from build123d import *

# Parameters (mm, degrees)
SKETCH2_W           = 1.5
SKETCH2_H           = 28.42
FILLET1_R           = 10
FILLET2_R           = 10
BOSS_EXTRUDE4_START = -11.350833333
BOSS_EXTRUDE4_DEPTH = 1
CIRPATTERN2_COUNT   = 6


with BuildPart() as part:
    # Sketch2 → Revolve1 (revolve)
    with BuildSketch(Plane(origin=(0, 0, 0), x_dir=(1, 0, 0), z_dir=(0, 1, 0))):
        with Locations((-5.020833333, 24.560833333)):
            Rectangle(SKETCH2_W, SKETCH2_H)
        with BuildLine():
            Line((-2.520833333, 11.350833333), (-4.020833333, 11.350833333))
            Line((-4.020833333, 11.350833333), (-4.020833333, -3.645335915))
            ThreePointArc((-4.020833333, -3.645335915), (-4.014018155, -3.844339123), (-4.020833333, -4.043342332))
            Line((-4.020833333, -4.043342332), (-4.020833333, -5.649166667))
            Line((-4.020833333, -5.649166667), (-2.520833333, -5.649166667))
            Line((-2.520833333, -5.649166667), (-2.520833333, 11.350833333))
        make_face()
        with BuildLine():
            Line((-2.520833333, -7.649166667), (-2.520833333, -5.649166667))
            Line((-2.520833333, -5.649166667), (-4.020833333, -5.649166667))
            Line((-4.020833333, -5.649166667), (-4.641637876, -5.649166667))
            ThreePointArc((-4.641637876, -5.649166667), (-6.922872715, -6.753193683), (-9.204107554, -5.649166667))
            Line((-9.204107554, -5.649166667), (-9.824912097, -5.649166667))
            Line((-9.824912097, -5.649166667), (-9.824912097, -7.649166667))
            Line((-9.824912097, -7.649166667), (-2.520833333, -7.649166667))
        make_face()
        with BuildLine():
            Line((-4.020833333, -5.649166667), (-4.020833333, -4.043342332))
            ThreePointArc((-4.020833333, -4.043342332), (-4.209710195, -4.893235682), (-4.641637876, -5.649166667))
            Line((-4.641637876, -5.649166667), (-4.020833333, -5.649166667))
        make_face()
        with BuildLine():
            Line((-9.824912097, -5.649166667), (-9.204107554, -5.649166667))
            ThreePointArc((-9.204107554, -5.649166667), (-9.636035235, -4.893235682), (-9.824912097, -4.043342332))
            Line((-9.824912097, -4.043342332), (-9.824912097, -5.649166667))
        make_face()
    revolve(axis=Axis((16.729166667, 0, -8.305777899), (0, 0, 1)))

    # Fillet1
    # the kernel refuses this fillet: 10 mm, written as the material it takes off along each edge
    with BuildSketch(Plane(origin=(16.729166667, 0, -10.350833333), x_dir=(-1, 0, 0), z_dir=(0, 1, 0))) as fillet1_piece_1:
        with BuildLine():
            CenterArc((31, -5.267826876), FILLET1_R, 148.211669383, 31.788330617)
            Line((22.5, 0), (22.33, 0.105356538))
            ThreePointArc((22.33, 0.105356538), (21.75, 0.2), (21, 0.2))
            Line((21, 0.2), (20.8, 0))
            Line((20.8, 0), (20.8, -5.267826876))
            Line((20.8, -5.267826876), (21, -5.267826876))
        make_face()
    revolve(axis=Axis((16.729166667, 0, -10.350833333), (0, 0, 1)), mode=Mode.SUBTRACT)

    # Fillet2
    # the kernel refuses this fillet: 10 mm, written as the material it takes off along each edge
    with BuildSketch(Plane(origin=(16.729166667, 0, -11.350833333), x_dir=(-1, 0, 0), z_dir=(0, 1, 0))) as fillet2_piece_1:
        with BuildLine():
            CenterArc((10.75, 5.267826876), FILLET2_R, 328.211669383, 31.788330617)
            Line((19.25, 0), (19.42, -0.105356538))
            ThreePointArc((19.42, -0.105356538), (20, -0.2), (20.75, -0.2))
            Line((20.75, -0.2), (20.95, 0))
            Line((20.95, 0), (20.95, 5.267826876))
            Line((20.95, 5.267826876), (20.75, 5.267826876))
        make_face()
    revolve(axis=Axis((16.729166667, 0, -11.350833333), (0, 0, 1)), mode=Mode.SUBTRACT)

    # Boss-Extrude4: read off the stored shape, not the designer's step
    # Boss-Extrude4 outline → Boss-Extrude4 (add)
    with BuildSketch(Plane.XY.offset(BOSS_EXTRUDE4_START)):
        with BuildLine():
            ThreePointArc((39.147683304, 1.913141856), (39.09932169, 2.413744857), (39.039783075, 2.913141856))
            Line((39.039783075, 2.913141856), (35.757464135, 2.913141856))
            ThreePointArc((35.757464135, 2.913141856), (35.827209818, 2.4139693), (35.883862912, 1.913141856))
            Line((35.883862912, 1.913141856), (39.147683304, 1.913141856))
        make_face()
    boss_extrude4 = extrude(amount=BOSS_EXTRUDE4_DEPTH)

    # CirPattern2: Boss-Extrude4 ×6 about axis
    cirpattern2_axis = Axis((16.729166667, 0, 0), (0, 0, 1))
    for i in range(1, CIRPATTERN2_COUNT):
        add(boss_extrude4.rotate(cirpattern2_axis, i * 360 / CIRPATTERN2_COUNT))


solid = part.part
Work out the finished part from the listing and answer in its coordinate system (mm). A direction names the side the tool comes from. Give positions to 0.01 mm unless a question says otherwise; leave off trailing zeros. Loops run counter-clockwise (first coordinate to the right, second up) from the corner with the lowest first, then second, coordinate; pieces in that order, holes last. Notation, with made-up numbers: (67, -15.5) -> (123, -15.5) arc R35 cw to (123, 20.5) -> close; hole circle Ø6 at (63, 10.25). An arc over 180 degrees is marked (long way). Use a Markdown table: item, result. Add a question column.
1) Each of these flat-tipped pins is pushed along its axis until it touches: P1, Ø1.1, axis at x = 29, y = -16, coming from the -Z side; P2, Ø1, axis at x = -1.5, z = -26.5, coming from the +Y side; P3, Ø0.8, axis at x = -4.5, z = -11, coming from the -Y side; P4, Ø3, axis at x = 10.5, y = 15, coming from the +Z side. Where does it stop, or does it pass through?
2) Which of the six approach directions +Z, -Z, +X, -X, +Y, -Y give full straight-line access (tool end or side, diameter ignored) to faces 4 (the flat face through (4, 17, -10.351)), 5 (the flat face through (29, -17, -10.351)), 6 (the cylindrical face through (-3.3, -6.31, -27.36)), 7 (the flat face through (24, 20, -38.771)), 8 (the flat face through (25, 19, -11.351))?
3) The part is cut by section B-B, the plane y = -1. Count the separate pieces of the cut face and the enclosed holes in it, plus the area to 3 significant figures.
4) The part is cut by section A-A, the plane z = -27. Determine the outline of the cut face in (x, y), plus the area to 3 significant figures.
5) For a pull along X with two mould halves and no side action, classify faces 1 (the flat face through (8.3, -19.4, -10.351)), 2 (the cylindrical face through (-2.439, 7.947, -1.151)), 3 (the flat face through (3.86, 16.46, -10.86)) as +X half, -X half, draft (parallel to the pull), parting line (faces both ways), or undercut.
6) Consider line 1 along X through (y, z) = (0, -1.75); line 2 along X through (y, z) = (0, -33.25); line 3 along Z through (x, y) = (32.5, 17.5). Determine where each line is inside the solid, lowest interval first.
Reported:
| question | item | result |
|---|---|---|
| 1 | P1 | stops at z = -11.35 |
| 1 | P2 | stops at y = 13.85 |
| 1 | P3 | stops at y = -8.51 |
| 1 | P4 | passes through |
| 2 | face 4 | -X, +Y |
| 2 | face 5 | +X, -Y |
| 2 | face 6 | -Z |
| 2 | face 7 | -Z, +X, -X, +Y, -Y |
| 2 | face 8 | none |
| 3 | separate pieces | 4 |
| 3 | enclosed holes | 0 |
| 3 | area | 150 mm^2 |
| 4 | outline | circle Ø45 at (16.73, 0); hole circle Ø42 at (16.73, 0) |
| 4 | area | 205 mm^2 |
| 5 | face 1 | draft |
| 5 | face 2 | parting line |
| 5 | face 3 | undercut |
| 6 | line 1 | x = -4.02 to -2.52, 35.98 to 37.48 |
| 6 | line 2 | x = -5.77 to -4.27, 37.73 to 39.23 |
| 6 | line 3 | z = 6.75 to 7.65 |
